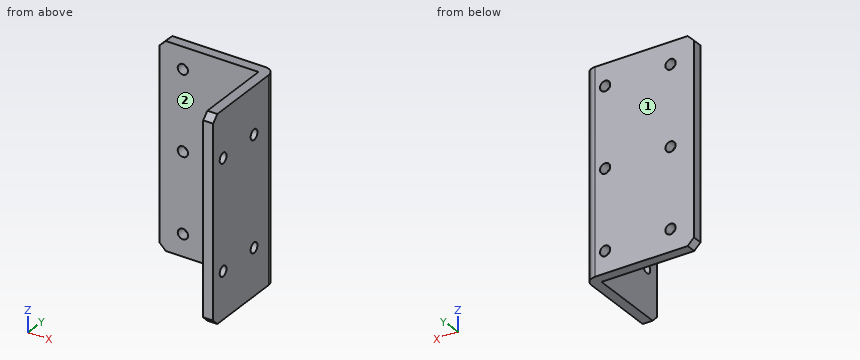
```python
from build123d import *

# Parameters (mm, degrees)
BOSS_EXTRUDE1_DEPTH       = 32.5
BOSS_EXTRUDE1_DEPTH_BACK  = 32.5
FILLET1_R                 = 3.2
M4X0_7_TAPPED_HOLE1_D     = 3.3
M4X0_7_TAPPED_HOLE1_DEPTH = 3.2
M4X0_7_TAPPED_HOLE2_D     = 3.3
M4X0_7_TAPPED_HOLE2_DEPTH = 3.2
LPATTERN1_COUNT           = 2
LPATTERN1_PITCH           = 21
LPATTERN1_COUNT_DIR2      = 3
LPATTERN1_PITCH_DIR2      = 25.5
CHAMFER1_SIZE             = 2


with BuildPart() as part:
    # Sketch1 → Boss-Extrude1 (new body, two sides)
    with BuildSketch(Plane.XY) as boss_extrude1_sk:
        Polygon((0, -30), (-3.2, -30), (-3.2, -3.2), (-35, -3.2), (-35, 0), (0, 0), align=None)
    extrude(amount=BOSS_EXTRUDE1_DEPTH)
    extrude(boss_extrude1_sk.sketch, amount=-BOSS_EXTRUDE1_DEPTH_BACK)

    # Fillet1
    fillet1_edges = [part.edges().sort_by_distance(p)[0] for p in [
        (0, 0, 0),
    ]]
    fillet(fillet1_edges, radius=FILLET1_R)

    # M4x0.7 Tapped Hole1
    with Locations(Plane(origin=(0, 0, 0), x_dir=(0, 0, -1), z_dir=(1, 0, 0))):
        with Locations((-17.5, -10.2), (-17.5, -25.2), (17.5, -25.2), (17.5, -10.2)):
            Hole(M4X0_7_TAPPED_HOLE1_D / 2, depth=M4X0_7_TAPPED_HOLE1_DEPTH)

    # M4x0.7 Tapped Hole2
    with Locations(Plane(origin=(0, 0, 0), x_dir=(-1, 0, 0), z_dir=(0, 1, 0))):
        with Locations((6.5, 25.5)):
            m4x0_7_tapped_hole2 = Hole(M4X0_7_TAPPED_HOLE2_D / 2, depth=M4X0_7_TAPPED_HOLE2_DEPTH)

    # LPattern1: M4x0.7 Tapped Hole2 2 × 3
    with Locations(*[(-i * LPATTERN1_PITCH, 0, -j * LPATTERN1_PITCH_DIR2) for i in range(LPATTERN1_COUNT) for j in range(LPATTERN1_COUNT_DIR2) if (i, j) != (0, 0)]):
        add(m4x0_7_tapped_hole2, mode=Mode.SUBTRACT)

    # Chamfer1
    chamfer1_edges = [part.edges().sort_by_distance(p)[0] for p in [
        (-35, -1.6, -32.5),
        (-35, -1.6, 32.5),
        (-1.6, -30, -32.5),
        (-1.6, -30, 32.5),
    ]]
    chamfer(chamfer1_edges, length=CHAMFER1_SIZE)


solid = part.part
```
Geometry check sheet. Reference: the model listing, model coordinates, mm. Face numbers are marked on the shaded views. A direction names the side the tool comes from. Round coordinates to 2 decimals unless told otherwise and drop trailing zeros. Order: outer loops, then holes, each group sorted by start corner. A loop starts at its lowest first (then second) coordinate and runs counter-clockwise, first axis right, second up. Notation, with made-up numbers: M -18.75,10.5 L -9.75,10.5 A7 cw -9.75,22.5 Z; hole C 21,72.5 d1. An arc over 180 degrees is marked long. Answer as CSV lines item,"result".
1) Sectioned sample at C-C on x = -6.5. Record the cut outline in (y, z), and give its area (3 significant figures).
Entries:
outline,"M -3.2,-32.5 L 0,-32.5 L 0,-27.15 L -3.2,-27.15 Z; M -3.2,-23.85 L 0,-23.85 L 0,-1.65 L -3.2,-1.65 Z; M -3.2,1.65 L 0,1.65 L 0,23.85 L -3.2,23.85 Z; M -3.2,27.15 L 0,27.15 L 0,32.5 L -3.2,32.5 Z"
area,"176 mm2"
2) Sectioned sample at B-B on y = -10.2. Record the cut outline in (x, z), and give its area (3 significant figures).
Entries:
outline,"M -3.2,-32.5 L 0,-32.5 L 0,-19.15 L -3.2,-19.15 Z; M -3.2,-15.85 L 0,-15.85 L 0,15.85 L -3.2,15.85 Z; M -3.2,19.15 L 0,19.15 L 0,32.5 L -3.2,32.5 Z"
area,"187 mm2"
3) Thickness scan on probe 1 along Z at (x, y) = (-27.5, -1.7); probe 2 along Y at (x, z) = (-1.6, -17.5); probe 3 along X at (y, z) = (-18, -25.5). Record the ranges inside material, lowest first. Write a range as [from, to].
Entries:
probe 1,"[-32.5, -27.15], [-23.85, -1.65], [1.65, 23.85], [27.15, 32.5]"
probe 2,"[-30, -26.85], [-23.55, -11.85], [-8.55, -0.43]"
probe 3,"[-3.2, 0]"
4) Sectioned sample at A-A on z = -17.5. Record the cut outline in (x, y).
Entries:
outline,"M -35,-3.2 L -3.2,-3.2 L -3.2,-8.55 L 0,-8.55 L 0,-3.2 A3.2 ccw -3.2,0 L -35,0 Z; M -3.2,-30 L 0,-30 L 0,-26.85 L -3.2,-26.85 Z; M -3.2,-23.55 L 0,-23.55 L 0,-11.85 L -3.2,-11.85 Z"
5) Tool access check on the marked faces 1 and 2. Record the directions out of +Z, -Z, +X, -X, +Y, -Y that give a thin tool (end or side, any length) a straight path to the whole face; none if there is none.
Entries:
face 1,"+Z, -Z, +X, -X, +Y"
face 2,"+Z, -Z, -X, -Y"
6) Gauge pin test, flat ends, axial feed: pin 1 Ø5.5 at (y, z) = (-25.2, 17.5) entering from -X; pin 2 Ø10 at (x, z) = (-27, 13.5) entering from +Y; pin 3 Ø4 at (x, z) = (-6.5, -25.5) entering from -Y. Record the tip position at first contact, or that the pin passes through.
Entries:
pin 1,"x = -3.2"
pin 2,"y = 0"
pin 3,"y = -3.2"
7) Sectioned sample at D-D on y = -26. Record the cut outline in (x, z), and give its area (3 significant figures).
Entries:
outline,"M -3.2,-32.5 L 0,-32.5 L 0,-18.94 L -3.2,-18.94 Z; M -3.2,-16.06 L 0,-16.06 L 0,16.06 L -3.2,16.06 Z; M -3.2,18.94 L 0,18.94 L 0,32.5 L -3.2,32.5 Z"
area,"190 mm2"
